Geometry check sheet. Reference: the model listing, model coordinates, mm. Face numbers are marked on the shaded views. A direction names the side the tool comes from. Give positions to 0.01 mm unless a question says otherwise; leave off trailing zeros. Write each loop counter-clockwise with the first axis right and the second up, starting at its lowest first coordinate (ties: lowest second). Pieces come first, ordered by that corner, then holes. Notation, with made-up numbers: M -6,64.25 L 2,64.25 A17 cw 2,92.25 Z; hole C 61,4 d5. An arc over 180 degrees is marked long. One line per item, written item: value. Start each with the question number.
1. Cross-section at A-A on y = 6.25. Record the cut outline in (x, z).
2. Cross-section at B-B on z = 10.25. Record the cut outline in (x, y), then the cut area to 3 significant figures.
3. Cross-section at D-D on z = 6. Record the cut outline in (x, y), then the cut area to 3 significant figures.
4. Scan lines: line 1 (Y direction, x = -9, z = 7.5); line 2 (X direction, y = 6.25, z = 4.25); line 3 (Z direction, x = -2.25, y = 0.5). Record each from-to range of solid material in increasing order.
5. Tool access check on the marked faces 4 and 5. Record the directions out of +Z, -Z, +X, -X, +Y, -Y that give a thin tool (end or side, any length) a straight path to the whole face; none if there is none.
6. Release check for a two-part mould opening along X. For the marked faces 1, 2 and 3 record: pulls with the +X half, pulls with the -X half, needs draft (parallel to the pull), parting line crosses it, or undercut.
7. Cross-section at C-C on y = 4.5. Record the cut outline in (x, z).
8. Gauge pin test, flat ends, axial feed: pin 1 (6.5 mm diameter, centred on y = 1, z = 9, fed in from -X); pin 2 (1.1 mm diameter, centred on y = -6, z = 5, fed in from +X); pin 3 (1.5 mm diameter, centred on x = -2, z = 2.5, fed in from +Y). Record the tip position at first contact, or that the pin passes through.
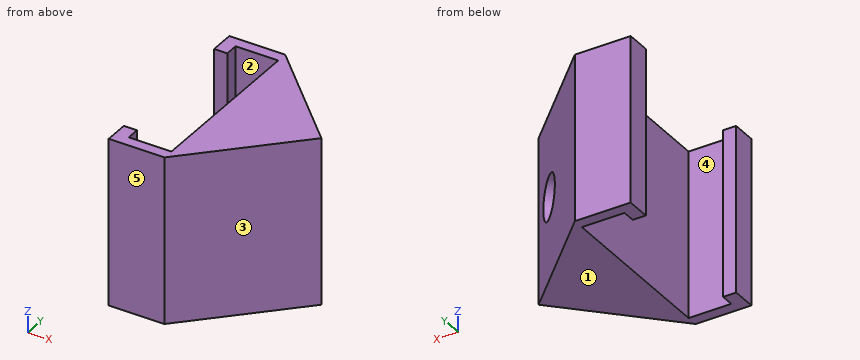
from build123d import *

# Parameters (mm, degrees)
BOSS_EXTRUDE1_DEPTH = 12.7
SKETCH7_R           = 1.65
CUT_EXTRUDE2_DEPTH  = 5


with BuildPart() as part:
    # Sketch1 → Boss-Extrude1 (new body)
    with BuildSketch(Plane.XY):
        Polygon((-7.35, 7.35), (0, 0), (-7.35, -7.35), (-11.6, -7.35), (-11.6, -6.5), (-11.6, -5.5), (-10.6, -5.5), (-10.6, -6.5), (-7.35, -6.5), (-7.35, 6.5), (-10.6, 6.5), (-10.6, 5.5), (-11.6, 5.5), (-11.6, 6.5), (-11.6, 7.35), align=None)
    extrude(amount=BOSS_EXTRUDE1_DEPTH)

    # Sketch7 → Cut-Extrude2 (cut)
    with BuildSketch(Plane(origin=(0, 0, 0), x_dir=(0, 0, -1), z_dir=(0.7071067811865724, 0.7071067811865226, 0))):
        with Locations(Location((-6.35, 3, 0), (0, 0, 90))):
            Circle(SKETCH7_R)
    extrude(amount=-CUT_EXTRUDE2_DEPTH, mode=Mode.SUBTRACT)


solid = part.part
Report:
1. outline: M -11.6,0 L -10.6,0 L -10.6,12.7 L -11.6,12.7 Z; M -7.35,0 L -6.25,0 L -6.25,12.7 L -7.35,12.7 Z
2. outline: M -11.6,-7.35 L -7.35,-7.35 L 0,0 L -7.35,7.35 L -11.6,7.35 L -11.6,5.5 L -10.6,5.5 L -10.6,6.5 L -7.35,6.5 L -7.35,-6.5 L -10.6,-6.5 L -10.6,-5.5 L -11.6,-5.5 Z
2. area: 63.2 mm^2
3. outline: M -11.6,-7.35 L -7.35,-7.35 L 0,0 L -0.98,0.98 L -4.52,-2.55 L -6.8,-0.27 L -3.26,3.26 L -7.35,7.35 L -11.6,7.35 L -11.6,5.5 L -10.6,5.5 L -10.6,6.5 L -7.35,6.5 L -7.35,-6.5 L -10.6,-6.5 L -10.6,-5.5 L -11.6,-5.5 Z
3. area: 47.1 mm^2
4. line 1: y = -7.35 to -6.5, 6.5 to 7.35
4. line 2: x = -11.6 to -10.6, -7.35 to -6.25
4. line 3: z = 0 to 5.08, 7.62 to 12.7
5. face 4: +Z, -Z
5. face 5: +Z, -Z, +X, -X, -Y
6. face 1: needs draft
6. face 2: undercut
6. face 3: pulls with the +X half
7. outline: M -7.35,0 L -4.5,0 L -4.5,12.7 L -7.35,12.7 Z
8. pin 1: stops at x = -7.35
8. pin 2: stops at x = -5.45
8. pin 3: stops at y = 2.75
